Design review of the part built by this model. Coordinates are the model's own, in mm. Face numbers are marked on the shaded views. A direction names the side the tool comes from. Coordinates: 2 decimals unless noted, no trailing zeros. Write each loop counter-clockwise with the first axis right and the second up, starting at its lowest first coordinate (ties: lowest second). Pieces come first, ordered by that corner, then holes. Notation, with made-up numbers: M 50,23 L 106,23 A15 cw 106,45 Z; hole C -27.5,-8 d11. An arc over 180 degrees is marked long. Write item = value, one per line.
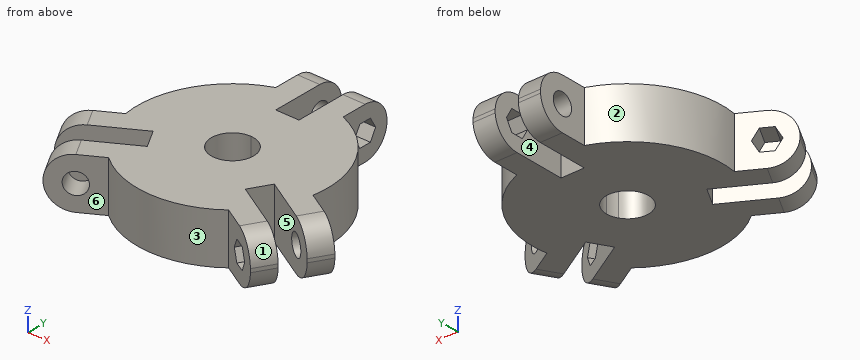
```python
from build123d import *

# Parameters (mm, degrees)
F1_DEPTH  = 12
F3_DEPTH  = 25
F5_DEPTH  = 25
F7_DEPTH  = 25
F8_R      = 2.5
F9_DEPTH  = 5.6
F11_DEPTH = 7
F12_R     = 2.5
F13_DEPTH = 7
F15_DEPTH = 7
F16_R     = 2.5
F17_DEPTH = 7
F19_DEPTH = 7


with BuildPart() as f1:
    # F0 (on Top) → F1 (new body)
    with BuildSketch(Plane.XY):
        with BuildLine():
            ThreePointArc((0, 5), (3.5355339059, 3.5355339059), (5, 0))
            ThreePointArc((5, 0), (4.8296291314, -1.2940952255), (4.3301270189, -2.5))
            Line((4.3301270189, -2.5), (12.9903810568, -7.5))
            Line((12.9903810568, -7.5), (14.3653810568, -5.1184301396))
            Line((14.3653810568, -5.1184301396), (29.9538383249, -14.1184301396))
            Line((29.9538383249, -14.1184301396), (32.5788383249, -9.5717967697))
            Line((32.5788383249, -9.5717967697), (22.2122898066, -3.5866671921))
            ThreePointArc((22.2122898066, -3.5866671921), (19.4855715851, 11.25), (8, 21.0297408448))
            Line((8, 21.0297408448), (8, 33))
            Line((8, 33), (2.75, 33))
            Line((2.75, 33), (2.75, 15))
            Line((2.75, 15), (0, 15))
            Line((0, 15), (0, 5))
        make_face()
        with BuildLine():
            ThreePointArc((-4.3301270189, -2.5), (-4.3301270189, 2.5), (0, 5))
            Line((0, 5), (0, 15))
            Line((0, 15), (-2.75, 15))
            Line((-2.75, 15), (-2.75, 33))
            Line((-2.75, 33), (-8, 33))
            Line((-8, 33), (-8, 21.0297408448))
            ThreePointArc((-8, 21.0297408448), (-19.4855715851, 11.25), (-22.2122898066, -3.5866671921))
            Line((-22.2122898066, -3.5866671921), (-32.5788383249, -9.5717967697))
            Line((-32.5788383249, -9.5717967697), (-29.9538383249, -14.1184301396))
            Line((-29.9538383249, -14.1184301396), (-14.3653810568, -5.1184301396))
            Line((-14.3653810568, -5.1184301396), (-12.9903810568, -7.5))
            Line((-12.9903810568, -7.5), (-4.3301270189, -2.5))
        make_face()
        with BuildLine():
            Line((12.9903810568, -7.5), (4.3301270189, -2.5))
            ThreePointArc((4.3301270189, -2.5), (0, -5), (-4.3301270189, -2.5))
            Line((-4.3301270189, -2.5), (-12.9903810568, -7.5))
            Line((-12.9903810568, -7.5), (-11.6153810568, -9.8815698604))
            Line((-11.6153810568, -9.8815698604), (-27.2038383249, -18.8815698604))
            Line((-27.2038383249, -18.8815698604), (-24.5788383249, -23.4282032303))
            Line((-24.5788383249, -23.4282032303), (-14.2122898066, -17.4430736527))
            ThreePointArc((-14.2122898066, -17.4430736527), (0, -22.5), (14.2122898066, -17.4430736527))
            Line((14.2122898066, -17.4430736527), (24.5788383249, -23.4282032303))
            Line((24.5788383249, -23.4282032303), (27.2038383249, -18.8815698604))
            Line((27.2038383249, -18.8815698604), (11.6153810568, -9.8815698604))
            Line((11.6153810568, -9.8815698604), (12.9903810568, -7.5))
        make_face()
    extrude(amount=F1_DEPTH)

    # F2 (on face) → F3 (cut)
    with BuildSketch(Plane(origin=(-8, 0, 0), x_dir=(0, -1, 0), z_dir=(-1, 0, 0))):
        with BuildLine():
            ThreePointArc((-27.0148704224, 0), (-31.1055308437, 1.6106381651), (-33, 5.5778342276))
            Line((-33, 5.5778342276), (-33, 0))
            Line((-33, 0), (-27.0148704224, 0))
        make_face()
        with BuildLine():
            Line((-33, 5.5778342276), (-33, 6.4221657724))
            ThreePointArc((-33, 6.4221657724), (-33.0148704224, 6), (-33, 5.5778342276))
        make_face()
        with BuildLine():
            ThreePointArc((-33, 6.4221657724), (-31.1055308437, 10.3893618349), (-27.0148704224, 12))
            Line((-27.0148704224, 12), (-33, 12))
            Line((-33, 12), (-33, 6.4221657724))
        make_face()
    extrude(amount=-F3_DEPTH, mode=Mode.SUBTRACT)

    # F4 (on face) → F5 (cut)
    with BuildSketch(Plane(origin=(-4, 6.9282032303, 0), x_dir=(-0.8660254038, -0.5, 0), z_dir=(-0.5, 0.8660254038, 0))):
        with BuildLine():
            Line((33, 12), (27.0148704224, 12))
            ThreePointArc((27.0148704224, 12), (31.1055308437, 10.3893618349), (33, 6.4221657724))
            Line((33, 6.4221657724), (33, 12))
        make_face()
        with BuildLine():
            Line((33, 0), (33, 5.5778342276))
            ThreePointArc((33, 5.5778342276), (31.1055308437, 1.6106381651), (27.0148704224, 0))
            Line((27.0148704224, 0), (33, 0))
        make_face()
        with BuildLine():
            ThreePointArc((33, 5.5778342276), (33.0148704224, 6), (33, 6.4221657724))
            Line((33, 6.4221657724), (33, 5.5778342276))
        make_face()
    extrude(amount=-F5_DEPTH, mode=Mode.SUBTRACT)

    # F6 (on face) → F7 (cut)
    with BuildSketch(Plane(origin=(-4, -6.9282032303, 0), x_dir=(0.8660254038, -0.5, 0), z_dir=(-0.5, -0.8660254038, 0))):
        with BuildLine():
            Line((33, 12), (27.0148704224, 12))
            ThreePointArc((27.0148704224, 12), (31.1055308437, 10.3893618349), (33, 6.4221657724))
            Line((33, 6.4221657724), (33, 12))
        make_face()
        with BuildLine():
            Line((33, 0), (33, 5.5778342276))
            ThreePointArc((33, 5.5778342276), (31.1055308437, 1.6106381651), (27.0148704224, 0))
            Line((27.0148704224, 0), (33, 0))
        make_face()
        with BuildLine():
            ThreePointArc((33, 5.5778342276), (33.0148704224, 6), (33, 6.4221657724))
            Line((33, 6.4221657724), (33, 5.5778342276))
        make_face()
    extrude(amount=-F7_DEPTH, mode=Mode.SUBTRACT)

    # F8 (on face) → F9 (cut)
    with BuildSketch(Plane(origin=(4, -6.9282032303, 0), x_dir=(0.8660254038, 0.5, 0), z_dir=(0.5, -0.8660254038, 0))):
        with Locations((-27.0148704224, 6)):
            Circle(F8_R)
    extrude(amount=-F9_DEPTH, mode=Mode.SUBTRACT)

    # F10 (on face) → F11 (cut)
    with BuildSketch(Plane(origin=(-4, 6.9282032303, 0), x_dir=(-0.8660254038, -0.5, 0), z_dir=(-0.5, 0.8660254038, 0))):
        Polygon((28.4582460954, 8.5), (25.5714947494, 8.5), (24.1281190765, 6), (25.5714947494, 3.5), (28.4582460954, 3.5), (29.9016217684, 6), align=None)
    extrude(amount=-F11_DEPTH, mode=Mode.SUBTRACT)

    # F12 (on face) → F13 (cut)
    with BuildSketch(Plane(origin=(-8, 0, 0), x_dir=(0, -1, 0), z_dir=(-1, 0, 0))):
        with Locations((-27.0148704224, 6)):
            Circle(F12_R)
    extrude(amount=-F13_DEPTH, mode=Mode.SUBTRACT)

    # F14 (on face) → F15 (cut)
    with BuildSketch(Plane.YZ.offset(8)):
        Polygon((28.4582460954, 8.5), (25.5714947494, 8.5), (24.1281190765, 6), (25.5714947494, 3.5), (28.4582460954, 3.5), (29.9016217684, 6), align=None)
    extrude(amount=-F15_DEPTH, mode=Mode.SUBTRACT)

    # F16 (on face) → F17 (cut)
    with BuildSketch(Plane(origin=(4, 6.9282032303, 0), x_dir=(-0.8660254038, 0.5, 0), z_dir=(0.5, 0.8660254038, 0))):
        with Locations((-27.0148704224, 6)):
            Circle(F16_R)
    extrude(amount=-F17_DEPTH, mode=Mode.SUBTRACT)

    # F18 (on face) → F19 (cut)
    with BuildSketch(Plane(origin=(-4, -6.9282032303, 0), x_dir=(0.8660254038, -0.5, 0), z_dir=(-0.5, -0.8660254038, 0))):
        Polygon((28.4582460954, 8.5), (25.5714947494, 8.5), (24.1281190765, 6), (25.5714947494, 3.5), (28.4582460954, 3.5), (29.9016217684, 6), align=None)
    extrude(amount=-F19_DEPTH, mode=Mode.SUBTRACT)


solid = f1.part
```
Q1. For P1, Ø1, axis at x = 12.5, y = 0.5, coming from the -Z side; P2, Ø5, axis at y = 21.5, z = 6, coming from the -X side; P3, Ø6, axis at x = -11, z = 4, coming from the -Y side; P4, Ø1.6, axis at x = -0.5, z = 4.5, coming from the +Y side, all flat-tipped, find the tip position at first contact; note any pin that passes through.
Check result:
P1 = 0
P2 = -12.05
P3 = -21.03
P4 = 15
Q2. The part is to be moulded in two halves that separate along X. For the marked faces 1, 2 and 3, say which applies: +X half, -X half, draft (parallel to the pull), parting line (faces both ways), or undercut.
Check result:
face_1 = +X half
face_2 = -X half
face_3 = undercut
Q3. Consider section B-B, the plane z = 10. State the section outline as (x, y) points, and give its area (3 significant figures).
Check result:
outline = M -31.27,-8.82 L -28.64,-13.36 L -14.37,-5.12 L -11.62,-9.88 L -25.89,-18.13 L -23.27,-22.67 L -14.21,-17.44 A22.5 ccw 14.21,-17.44 L 23.27,-22.67 L 25.89,-18.13 L 11.62,-9.88 L 14.37,-5.12 L 28.64,-13.36 L 31.27,-8.82 L 22.21,-3.59 A22.5 ccw 8,21.03 L 8,31.49 L 2.75,31.49 L 2.75,15 L -2.75,15 L -2.75,31.49 L -8,31.49 L -8,21.03 A22.5 ccw -22.21,-3.59 Z; hole C 0,0 d10
area = 1,690 mm²
Q4. Machinability: for the marked faces 4, 5 and 6, which of the approach directions +Z, -Z, +X, -X, +Y, -Y give a long, thin tool a straight path to every point of the face, cutting with its end or side? Answer none if there is none.
Check result:
face_4 = +Z, -Z, +Y
face_5 = +Z, -Z
face_6 = +Z, -Z, -Y
Q5. Wall thickness on line 1 (X direction, y = -20, z = 6.25); line 2 (X direction, y = -6, z = 2); line 3 (X direction, y = 21.5, z = 3.5): over which ranges is each line inside the solid? List them lowest first.
Check result:
line_1 = -26.56 to -22.52, -10.31 to 10.31, 22.81 to 26.56
line_2 = -26.39 to -15.89, -13.86 to 13.86, 15.89 to 26.39
line_3 = -8 to -2.75, 2.75 to 8
Q6. Consider section C-C, the plane z = 2.75. State the section outline as (x, y) points.
Check result:
outline = M -31.76,-9.1 L -29.14,-13.65 L -14.37,-5.12 L -11.62,-9.88 L -26.39,-18.41 L -23.76,-22.96 L -14.21,-17.44 A22.5 ccw 14.21,-17.44 L 23.76,-22.96 L 26.39,-18.41 L 11.62,-9.88 L 14.37,-5.12 L 29.14,-13.65 L 31.76,-9.1 L 22.21,-3.59 A22.5 ccw 8,21.03 L 8,32.06 L 2.75,32.06 L 2.75,15 L -2.75,15 L -2.75,32.06 L -8,32.06 L -8,21.03 A22.5 ccw -22.21,-3.59 Z; hole C 0,0 d10
Q7. Consider section A-A, the plane x = 7. State the section outline as (y, z) points.
Check result:
outline = M -21.38,0 L 27.01,0 A6 ccw 33,5.58 L 33,6.42 A6 ccw 27.01,12 L -21.38,12 Z; hole M 24.13,6 L 25.57,3.5 L 28.46,3.5 L 29.9,6 L 28.46,8.5 L 25.57,8.5 Z
